```python
from build123d import *

# Parameters (mm, degrees)
F0_W   = 0.2
F0_H   = 1.1
F0_W_2 = 0.8
F0_H_2 = 1.5


# Not quite as in the source:
# - a feature names something its author has since deleted; it is built from what else it names


with BuildPart() as f1:
    # F0 (on Front) → F1 (revolve)
    with BuildSketch(Plane.XZ):
        Polygon((4.71, 2.6), (0, 2.6), (0, 1.5), (1.21, 1.5), (2.01, 1.5), (3.91, 1.5), (3.91, 1.1), (3.91, 0), (4.71, 0), (4.71, 1.1), align=None)
        with Locations((4.81, 0.55)):
            Rectangle(F0_W, F0_H)
        with Locations((3.81, 0.55)):
            Rectangle(F0_W, F0_H)
        with Locations((1.61, 0.75)):
            Rectangle(F0_W_2, F0_H_2)
    revolve(axis=Axis((0, 0, 1.3), (0, 0, 1)))


solid = f1.part
```
For this review, take the finished solid that the model builds, in its own axes (mm). A direction names the side the tool comes from. Round coordinates to 2 decimals unless told otherwise and drop trailing zeros. Write each loop counter-clockwise with the first axis right and the second up, starting at its lowest first coordinate (ties: lowest second). Pieces come first, ordered by that corner, then holes. Notation, with made-up numbers: (-0.75, -27.5) - (39.25, -27.5) arc R22 ccw to (39.25, 8.5) - close; hole circle Ø6 at (-5.75, 62.25). An arc over 180 degrees is marked (long way). Put each result on its own line as item: value.
Q1. Machinability: for faces 4 (the face through (1.081, 1.695, 0.76)), 5 (the face through (-1.02, -4.6, 1.86)), 6 (the face through (-1, -1, 0)), 7 (the face through (3.73, 1.17, 1.3)), which of the approach directions +Z, -Z, +X, -X, +Y, -Y give a long, thin tool a straight path to every point of the face, cutting with its end or side? Answer none if there is none.
Solved:
face 4: -Z
face 5: +Z
face 6: -Z, +X, -X, +Y, -Y
face 7: none
Q2. Mouldability with a two-part tool opening along X and no side actions: class faces 1 (the face through (0, 0, 2.6)), 2 (the face through (0, 0, 1.5)), 3 (the face through (4.683, 1.475, 0.558)) as released by +X, released by -X, zero draft, split by the parting line, or undercut.
Solved:
face 1: zero draft
face 2: undercut
face 3: split by the parting line
Q3. We need section A-A (z = 0.2). Give the boundary of the cut face in (x, y), and give its area (3 significant figures).
Solved:
outline: circle Ø9.82 at (0, 0); circle Ø4.02 at (0, 0); hole circle Ø7.42 at (0, 0); hole circle Ø2.42 at (0, 0)
area: 40.6 mm2
Q4. We need section B-B (x = 0). Give the boundary of the cut face in (y, z).
Solved:
outline: (-4.91, 0) - (-3.71, 0) - (-3.71, 1.1) - (-3.91, 1.1) - (-3.91, 1.5) - (-2.01, 1.5) - (-2.01, 0) - (-1.21, 0) - (-1.21, 1.5) - (1.21, 1.5) - (1.21, 0) - (2.01, 0) - (2.01, 1.5) - (3.91, 1.5) - (3.91, 1.1) - (3.71, 1.1) - (3.71, 0) - (4.91, 0) - (4.91, 1.1) - (4.71, 1.1) - (4.71, 2.6) - (-4.71, 2.6) - (-4.71, 1.1) - (-4.91, 1.1) - close
Q5. Insertion check: pin 1 Ø1.5 at (y, z) = (2.5, 0.5) entering from -X; pin 2 Ø1.2 at (x, y) = (0.5, 0) entering from -Z. Each pin has a flat end and moves straight along its axis. Give the tip position at first contact, or say it passes through.
Solved:
pin 1: stops at x = -4.59
pin 2: stops at z = 1.5
Q6. Wall thickness on probe 1 along Y at (x, z) = (0, 1.25); probe 2 along Y at (x, z) = (0, 0.7); probe 3 along X at (y, z) = (-1.5, 0.3): over which ranges is each line inside the solid? List them lowest first.
Solved:
probe 1: y = -4.71 to -3.91, -2.01 to -1.21, 1.21 to 2.01, 3.91 to 4.71
probe 2: y = -4.91 to -3.71, -2.01 to -1.21, 1.21 to 2.01, 3.71 to 4.91
probe 3: x = -4.68 to -3.39, -1.34 to 1.34, 3.39 to 4.68
Q7. We need section C-C (z = 1.25). Give the boundary of the cut face in (x, y), and give its area (3 significant figures).
Solved:
outline: circle Ø9.42 at (0, 0); circle Ø4.02 at (0, 0); hole circle Ø7.82 at (0, 0); hole circle Ø2.42 at (0, 0)
area: 29.8 mm2
Q8. We need section D-D (y = -2.5). Give the boundary of the cut face in (x, z).
Solved:
outline: (-4.23, 0) - (-2.74, 0) - (-2.74, 1.1) - (-3.01, 1.1) - (-3.01, 1.5) - (3.01, 1.5) - (3.01, 1.1) - (2.74, 1.1) - (2.74, 0) - (4.23, 0) - (4.23, 1.1) - (3.99, 1.1) - (3.99, 2.6) - (-3.99, 2.6) - (-3.99, 1.1) - (-4.23, 1.1) - close
